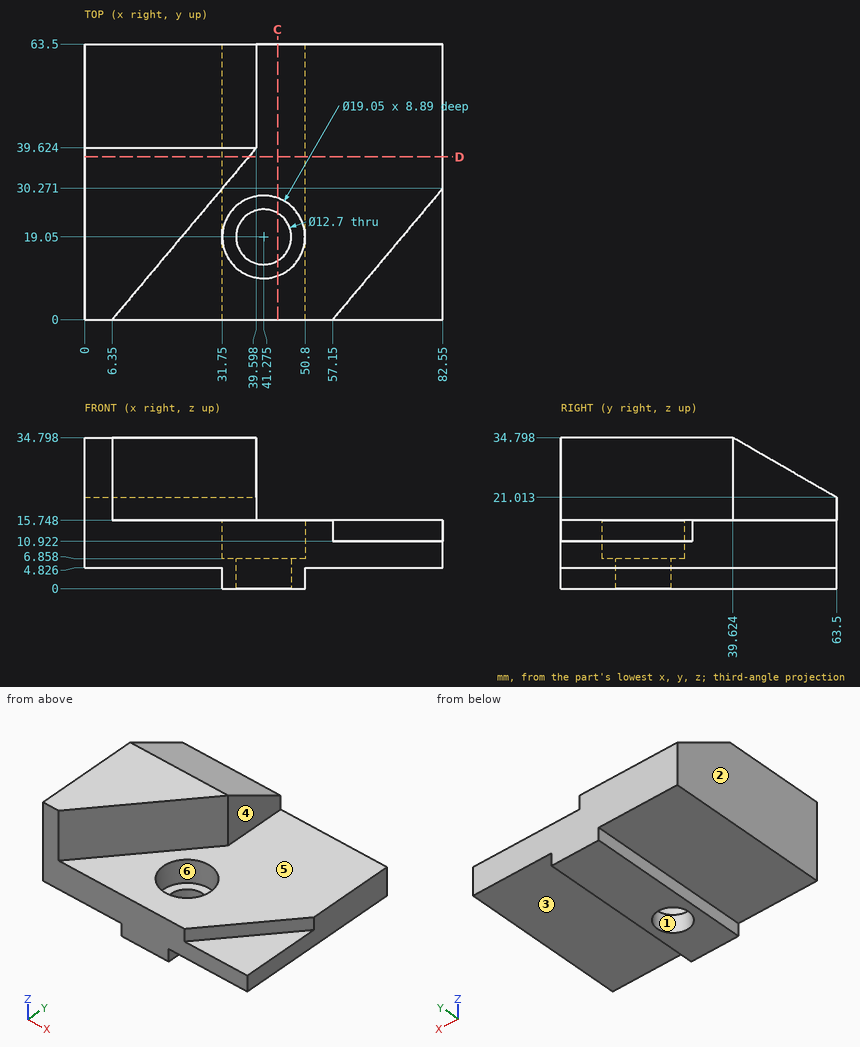
Input: dimensioned drawing with shaded views. Units: mm. Origin: part minimum x, y, z. A direction names the side the tool comes from. Coordinates: 2 decimals unless noted, no trailing zeros. Order: outer loops, then holes, each group sorted by start corner. A loop starts at its lowest first (then second) coordinate and runs counter-clockwise, first axis right, second up.
1. Draft query along X for the marked faces 1, 2 and 3. Return one class per face: +X half, -X half, draft (parallel to the pull), parting line (faces both ways), or undercut.
Checked values:
face 1: undercut
face 2: -X half
face 3: draft
2. Cut plane D-D, the plane y = 37.5. Return loops of the section in (x, z), plus the area to 3 significant figures.
Checked values:
outline: (0, 4.83) - (31.75, 4.83) - (31.75, 0) - (50.8, 0) - (50.8, 4.83) - (82.55, 4.83) - (82.55, 15.75) - (37.82, 15.75) - (37.82, 34.8) - (0, 34.8) - close
area: 1,710 mm2
3. Cut plane C-C, the plane x = 44.5. Return loops of the section in (y, z).
Checked values:
outline: (0, 0) - (13.58, 0) - (13.58, 6.86) - (10.09, 6.86) - (10.09, 15.75) - (0, 15.75) - close; (24.52, 0) - (63.5, 0) - (63.5, 15.75) - (28.01, 15.75) - (28.01, 6.86) - (24.52, 6.86) - close
4. Contact query for flat-ended pins moving along their axis: P1, Ø21, axis at x = 40.5, y = 19.5, coming from the +Z side; P2, Ø2, axis at y = 11, z = 22.5, coming from the +X side; P3, Ø1.4, axis at y = 42, z = 3, coming from the -X side. Output: stop coordinate, or through.
Checked values:
P1: stops at z = 15.75
P2: stops at x = 16.42
P3: stops at x = 31.75
5. Access query for the marked faces 4, 5 and 6. Directions: +Z, -Z, +X, -X, +Y, -Y. A direction counts if a zero-diameter tool reaches every point of the face in a straight line with its end or side. Return the directions, or none.
Checked values:
face 4: +Z, +X, +Y, -Y
face 5: +Z, +X, -Y
face 6: +Z
6. Ray query, line 1 along X through (y, z) = (19, 10); line 2 along Z through (x, y) = (70, 38); line 3 along Z through (x, y) = (27.5, 32). Return the intervals inside material, ascending.
Checked values:
line 1: x = 0 to 31.75, 50.8 to 82.55
line 2: z = 4.83 to 15.75
line 3: z = 4.83 to 34.8
